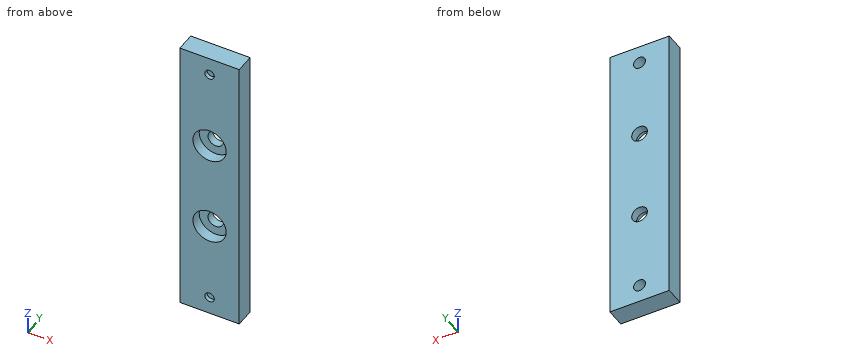
```python
from build123d import *

# Parameters (mm, degrees)
SKICA1_W                                          = 25
SKICA1_H                                          = 120
P_IDAT_VYSUNUT_M1_DEPTH                           = 8
D_RY_PRO_KOL_K_VELIKOST_MM2_D                     = 5
D_RY_PRO_KOL_K_VELIKOST_MM2_DEPTH                 = 6
D_RY_PRO_KOL_K_VELIKOST_MM2_2_D                   = 4
D_RY_PRO_KOL_K_VELIKOST_MM2_2_DEPTH               = 1.7
V_LCOV_ZAHLOUBEN_PRO_M6_ROUBY_S_V_LCO_D           = 6.6
V_LCOV_ZAHLOUBEN_PRO_M6_ROUBY_S_V_LCO_CBORE_D     = 14
V_LCOV_ZAHLOUBEN_PRO_M6_ROUBY_S_V_LCO_CBORE_DEPTH = 4.6


with BuildPart() as part:
    # Skica1 → Přidat vysunutím1 (new body)
    with BuildSketch(Plane(origin=(0, 0, 0), x_dir=(1, 0, 0), z_dir=(0, 1, 0))):
        Rectangle(SKICA1_W, SKICA1_H)
    extrude(amount=P_IDAT_VYSUNUT_M1_DEPTH)

    # D_ry pro kol_k_ velikost mm2
    with Locations(Plane(origin=(0, 8, 0), x_dir=(1, 0, 0), z_dir=(0, 1, 0))):
        with Locations((0, -52.5), (0, 52.5)):
            Hole(D_RY_PRO_KOL_K_VELIKOST_MM2_D / 2, depth=D_RY_PRO_KOL_K_VELIKOST_MM2_DEPTH)

    # D_ry pro kol_k_ velikost mm2 2
    with Locations(Plane(origin=(0, 0, 0), x_dir=(-1, 0, 0), z_dir=(0, -1, 0))):
        with Locations((0, -52.5), (0, 52.5)):
            Hole(D_RY_PRO_KOL_K_VELIKOST_MM2_2_D / 2, depth=D_RY_PRO_KOL_K_VELIKOST_MM2_2_DEPTH)

    # Válcové zahloubení pro M6 šrouby s válcovou hlavou zaoblenou1 (through all)
    with Locations(Plane(origin=(0, 0, 0), x_dir=(-1, 0, 0), z_dir=(0, -1, 0))):
        with Locations((0, -19), (0, 19)):
            CounterBoreHole(V_LCOV_ZAHLOUBEN_PRO_M6_ROUBY_S_V_LCO_D / 2, V_LCOV_ZAHLOUBEN_PRO_M6_ROUBY_S_V_LCO_CBORE_D / 2, V_LCOV_ZAHLOUBEN_PRO_M6_ROUBY_S_V_LCO_CBORE_DEPTH)


solid = part.part
```
The model under review builds one solid part; all positions refer to its coordinate system, in mm. Round coordinates to 2 decimals unless told otherwise and drop trailing zeros. Order: outer loops, then holes, each group sorted by start corner. A loop starts at its lowest first (then second) coordinate and runs counter-clockwise, first axis right, second up. Notation, with made-up numbers: M 7,-32.5 L 19,-32.5 A8 cw 19,-19.5 Z; hole C 66,22 d6. An arc over 180 degrees is marked long. Use a Markdown table: item, result.
1) Consider section C-C (x = 0). Give the number of separate pieces and of enclosed holes in the cut face, then the cut area to 3 significant figures.
Report:
| item | result |
|---|---|
| separate pieces | 3 |
| enclosed holes | 0 |
| area | 713 mm^2 |
2) Consider section D-D (z = -52.5). Write out the cut boundary in (x, y), then the cut area to 3 significant figures.
Report:
| item | result |
|---|---|
| outline | M -12.5,0 L -2,0 L -2,1.7 L 2,1.7 L 2,0 L 12.5,0 L 12.5,8 L 2.5,8 L 2.5,2 L -2.5,2 L -2.5,8 L -12.5,8 Z |
| area | 163 mm^2 |
3) Consider section A-A (y = 3). Write out the cut boundary in (x, z), then the cut area to 3 significant figures.
Report:
| item | result |
|---|---|
| outline | M -12.5,-60 L 12.5,-60 L 12.5,60 L -12.5,60 Z; hole C 0,-19 d14; hole C 0,19 d14; hole C 0,-52.5 d5; hole C 0,52.5 d5 |
| area | 2,650 mm^2 |
4) Insertion check: pin 1 (4.5 mm diameter, centred on x = 0, z = -52.5, fed in from -Y); pin 2 (1.5 mm diameter, centred on x = 0, z = -51.5, fed in from +Y); pin 3 (6 mm diameter, centred on x = 0, z = 19, fed in from +Y); pin 4 (1.2 mm diameter, centred on x = 0.5, z = -53, fed in from -Y). Each pin has a flat end and moves straight along its axis. Give the tip position at first contact, or say it passes through.
Report:
| item | result |
|---|---|
| pin 1 | y = 0 |
| pin 2 | y = 2 |
| pin 3 | through |
| pin 4 | y = 1.7 |
5) Consider section B-B (z = -19). Write out the cut boundary in (x, y).
Report:
| item | result |
|---|---|
| outline | M -12.5,0 L -7,0 L -7,4.6 L -3.3,4.6 L -3.3,8 L -12.5,8 Z; M 3.3,4.6 L 7,4.6 L 7,0 L 12.5,0 L 12.5,8 L 3.3,8 Z |
6) Wall thickness on line 1 along Z through (x, y) = (0, 1.35); line 2 along Z through (x, y) = (0, 3.7); line 3 along Z through (x, y) = (0, 1.85): over which ranges is each line inside the solid? List them lowest first. Write a range as [from, to].
Report:
| item | result |
|---|---|
| line 1 | [-60, -54.5], [-50.5, -26], [-12, 12], [26, 50.5], [54.5, 60] |
| line 2 | [-60, -55], [-50, -26], [-12, 12], [26, 50], [55, 60] |
| line 3 | [-60, -26], [-12, 12], [26, 60] |
